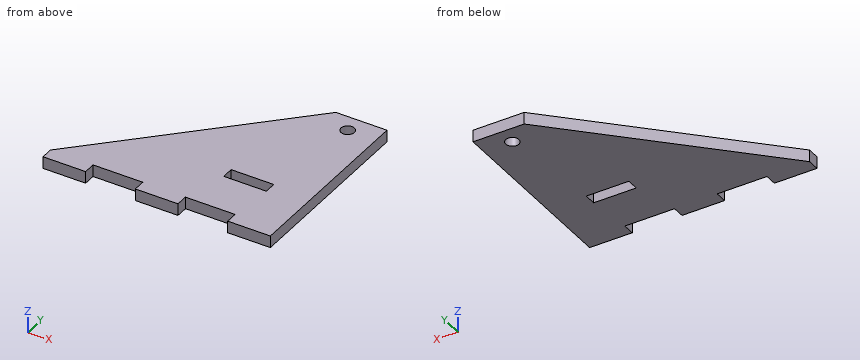
from build123d import *

# Parameters (mm, degrees)
BASE_DEPTH         = 5.334
SKETCH2_R          = 2.975
SKETCH2_W          = 19.05
SKETCH2_H          = 5.334
MOUNT_POINTS_DEPTH = 129.650686574
SKETCH3_W          = 19.05
SKETCH3_H          = 5.334
TABS_DEPTH         = 5.334


with BuildPart() as part:
    # Sketch1 → Base (new body)
    with BuildSketch(Plane.XY):
        Polygon((78.74, 78.74), (0, 0), (101.6, 0), (101.6, 78.74), align=None)
    extrude(amount=BASE_DEPTH)

    # Sketch2 → Mount Points (cut, through all)
    with BuildSketch(Plane.XY.offset(5.334)):
        with Locations((88.9, 70.866)):
            Circle(SKETCH2_R)
        with Locations((74.84, 22.256365646)):
            Rectangle(SKETCH2_W, SKETCH2_H)
    extrude(amount=-MOUNT_POINTS_DEPTH, mode=Mode.SUBTRACT)

    # Sketch3 → Tabs (add)
    with BuildSketch(Plane.XZ):
        with Locations((9.525, 2.667)):
            Rectangle(SKETCH3_W, SKETCH3_H)
        with Locations((92.075, 2.667)):
            Rectangle(SKETCH3_W, SKETCH3_H)
        with Locations((50.8, 2.667)):
            Rectangle(SKETCH3_W, SKETCH3_H)
    extrude(amount=TABS_DEPTH)


solid = part.part
Read the model definition and answer for the solid it produces. Units are mm, in the model's axes. Round coordinates to 2 decimals unless told otherwise and drop trailing zeros. Write each loop counter-clockwise with the first axis right and the second up, starting at its lowest first coordinate (ties: lowest second). Pieces come first, ordered by that corner, then holes.
Q1. Flat-ended cylindrical pins translate along their axes: P1, Ø2, axis at x = 69.5, z = 2, coming from the -Y side; P2, Ø2, axis at y = 43.5, z = 2, coming from the -X side; P3, Ø2.5, axis at x = 74.5, z = 2, coming from the +Y side. Find the tip coordinate at first contact, or state that the pin passes through.
Values:
P1: stops at y = 0
P2: stops at x = 42.5
P3: stops at y = 75.75
Q2. Find section A-A on x = 88.9. Determine the outline of the cut face in (y, z), and give its area (3 significant figures).
Values:
outline: (-5.33, 0) - (67.89, 0) - (67.89, 5.33) - (-5.33, 5.33) - close; (73.84, 0) - (78.74, 0) - (78.74, 5.33) - (73.84, 5.33) - close
area: 417 mm2
Q3. Straight lines are drawn through the part: line 1 (X direction, y = -0.5, z = 0.3) (3 decimals); line 2 (Y direction, x = 88.9, z = 1.65); line 3 (Y direction, x = 90.5, z = 4.1). For each, find the intervals that lie inside material, in ascending order.
Values:
line 1: x = 0 to 19.05, 41.275 to 60.325, 82.55 to 101.6
line 2: y = -5.33 to 67.89, 73.84 to 78.74
line 3: y = -5.33 to 68.36, 73.37 to 78.74
Q4. Find section C-C on z = 3.7. Determine the outline of the cut face in (x, y) (3 decimals), and give its area (3 significant figures).
Values:
outline: (0, -5.334) - (19.05, -5.334) - (19.05, 0) - (41.275, 0) - (41.275, -5.334) - (60.325, -5.334) - (60.325, 0) - (82.55, 0) - (82.55, -5.334) - (101.6, -5.334) - (101.6, 78.74) - (78.74, 78.74) - (0, 0) - close; hole (65.315, 19.589) - (84.365, 19.589) - (84.365, 24.923) - (65.315, 24.923) - close; hole circle Ø5.95 at (88.9, 70.866)
area: 5,080 mm2
Q5. Find section D-D on y = 12. Determine the outline of the cut face in (x, z).
Values:
outline: (12, 0) - (101.6, 0) - (101.6, 5.33) - (12, 5.33) - close
Q6. Find section B-B on y = 69.5. Determine the outline of the cut face in (x, z).
Values:
outline: (69.5, 0) - (86.26, 0) - (86.26, 5.33) - (69.5, 5.33) - close; (91.54, 0) - (101.6, 0) - (101.6, 5.33) - (91.54, 5.33) - close
